from build123d import *

# Parameters (mm, degrees)
BOSS_EXTRUDE1_DEPTH             = 30
CUT_EXTRUDE2_DEPTH              = 9.8
CBORE_FOR_M4_SBHCS1_D           = 4.5
CBORE_FOR_M4_SBHCS1_CBORE_D     = 8.6
CBORE_FOR_M4_SBHCS1_CBORE_DEPTH = 8
F_6_0_6_DIAMETER_HOLE1_D        = 6
SKETCH9_W                       = 7.5
SKETCH9_H                       = 8
CUT_EXTRUDE3_DEPTH              = 19
CUT_EXTRUDE3_DEPTH_BACK         = 19
CHAMFER1_SIZE2                  = 1.68681461
CHAMFER1_SIZE                   = 2
CHAMFER1_EDGE_2_SIZE2           = 1.68681461
CHAMFER1_EDGE_2_SIZE            = 2
F_7_5_7_5_DIAMETER_HOLE1_D      = 7.5
F_7_5_7_5_DIAMETER_HOLE1_DEPTH  = 7
F_7_5_7_5_DIAMETER_HOLE1_TIP    = 2.253227321


with BuildPart() as part:
    # Sketch1 → Boss-Extrude1 (new body)
    with BuildSketch(Plane(origin=(0, 0, 0), x_dir=(1, 0, 0), z_dir=(0, 1, 0))):
        Polygon((-18, 0), (18, 0), (18, 20.8), (14, 24.8), (-14, 24.8), (-18, 20.8), align=None)
    extrude(amount=BOSS_EXTRUDE1_DEPTH)

    # Sketch7 → Cut-Extrude2 (cut)
    with BuildSketch(Plane(origin=(0, 16, 0), x_dir=(1, 0, 0), z_dir=(0, 1, 0))):
        with BuildLine():
            Line((-7, 21.3), (7, 21.3))
            ThreePointArc((7, 21.3), (9.706928791, 20.34103824), (11.206489583, 17.891877451))
            Line((11.206489583, 17.891877451), (15, 0))
            Line((15, 0), (-15, 0))
            Line((-15, 0), (-11.206489583, 17.891877451))
            ThreePointArc((-11.206489583, 17.891877451), (-9.706928791, 20.34103824), (-7, 21.3))
        make_face()
    extrude(amount=CUT_EXTRUDE2_DEPTH, mode=Mode.SUBTRACT)

    # CBORE for M4 SBHCS1 (through all)
    with Locations(Plane(origin=(0, 30, 0), x_dir=(1, 0, 0), z_dir=(0, 1, 0))):
        with Locations((-7, 17), (7, 17)):
            CounterBoreHole(CBORE_FOR_M4_SBHCS1_D / 2, CBORE_FOR_M4_SBHCS1_CBORE_D / 2, CBORE_FOR_M4_SBHCS1_CBORE_DEPTH)

    # Ø6.0 (6) Diameter Hole1 (through all)
    with Locations(Plane(origin=(0, 30, 0), x_dir=(1, 0, 0), z_dir=(0, 1, 0))):
        with Locations((-7, 6), (7, 6)):
            Hole(F_6_0_6_DIAMETER_HOLE1_D / 2)

    # Sketch9 → Cut-Extrude3 (cut, two sides)
    with BuildSketch(Plane(origin=(0, 0, 0), x_dir=(0, 0, -1), z_dir=(1, 0, 0))) as cut_extrude3_sk:
        with Locations((13.75, 20)):
            Rectangle(SKETCH9_W, SKETCH9_H)
    extrude(amount=CUT_EXTRUDE3_DEPTH, mode=Mode.SUBTRACT)
    extrude(cut_extrude3_sk.sketch, amount=-CUT_EXTRUDE3_DEPTH_BACK, mode=Mode.SUBTRACT)

    # Chamfer1
    chamfer1_edges = [part.edges().sort_by_distance(p)[0] for p in [
        (-12.879758328, 20, -10),
    ]]
    chamfer(chamfer1_edges, length=CHAMFER1_SIZE, length2=CHAMFER1_SIZE2)

    # Chamfer1 edge 2
    chamfer1_edge_2_edges = [part.edges().sort_by_distance(p)[0] for p in [
        (12.879758328, 20, -10),
    ]]
    chamfer(chamfer1_edge_2_edges, length=CHAMFER1_EDGE_2_SIZE, length2=CHAMFER1_EDGE_2_SIZE2)

    # Ø7.5 (7.5) Diameter Hole1
    with Locations(Plane(origin=(0, 30, 0), x_dir=(1, 0, 0), z_dir=(0, 1, 0))):
        with Locations((-7, 6), (7, 6)):
            Hole(F_7_5_7_5_DIAMETER_HOLE1_D / 2, depth=F_7_5_7_5_DIAMETER_HOLE1_DEPTH)
            with Locations((0, 0, -(F_7_5_7_5_DIAMETER_HOLE1_DEPTH + F_7_5_7_5_DIAMETER_HOLE1_TIP / 2))):  # 118° drill point
                Cone(0, F_7_5_7_5_DIAMETER_HOLE1_D / 2, F_7_5_7_5_DIAMETER_HOLE1_TIP, mode=Mode.SUBTRACT)


solid = part.part
Design review of the part built by this model. Coordinates are the model's own, in mm. A direction names the side the tool comes from. Give positions to 0.01 mm unless a question says otherwise; leave off trailing zeros. Loops run counter-clockwise (first coordinate to the right, second up) from the corner with the lowest first, then second, coordinate; pieces in that order, holes last. Notation, with made-up numbers: M 60,2 L 92,2 A23 cw 92,13 Z; hole C 33,78 d5. An arc over 180 degrees is marked long. One line per question, with ' | ' between items. Start each with the question number.
1. Add section B-B (z = -16.5). Write out the cut boundary in (x, y), plus the area to 3 significant figures.
2. To check wall thickness, follow L1, parallel to X at y = 7.25, z = -17; L2, parallel to X at y = 26, z = -17; L3, parallel to Z at x = 7, y = 5.75. State the ranges of each line that lie inside material, in increasing order.
3. Insertion check: P1, Ø1, axis at x = -8.5, z = -17.5, coming from the +Y side; P2, Ø7, axis at x = -7, z = -6, coming from the +Y side; P3, Ø1, axis at x = 16, y = 22, coming from the -Z side. Each pin has a flat end and moves straight along its axis. Give the tip position at first contact, or say it passes through.
4. The part is to be moulded in two halves that separate along Y. For faces 1 (the face through (0, 30, -13)), 2 (the face through (0, 16, -11)), 3 (the face through (-9.77, 7.89, -4.85)), say which applies: released by +Y, released by -Y, zero draft, split by the parting line, or undercut.
5. For faces 4 (the face through (-13.973, 21.92, -4.845)), 5 (the face through (0, 15, -24.8)), 6 (the face through (15, 20, -17.5)), 7 (the face through (9.976, 27.871, -3.718)), 8 (the face through (-13.939, 20.056, -9.035)), list the 3-axis set-ups (+Z, -Z, +X, -X, +Y, -Y) from which the entire face can be reached by the end or side of a thin tool; tool diameter is ignored.
6. Add section C-C (x = 8). Write out the cut boundary in (y, z).
7. Add section A-A (y = 17.5). Write out the cut boundary in (x, z).
8. Add section D-D (y = 12.25). Write out the cut boundary in (x, z), plus the area to 3 significant figures.
Worked out:
1) outline: M -18,0 L -9.19,0 L -9.19,16 L -18,16 Z; M -18,24 L -11.5,24 L -11.5,25.8 L -11.27,25.8 L -11.27,30 L -18,30 Z; M -4.81,0 L 4.81,0 L 4.81,16 L -4.81,16 Z; M -2.73,25.8 L 2.73,25.8 L 2.73,30 L -2.73,30 Z; M 9.19,0 L 18,0 L 18,16 L 9.19,16 Z; M 11.27,25.8 L 11.5,25.8 L 11.5,24 L 18,24 L 18,30 L 11.27,30 Z | area: 538 mm²
2) L1: x = -18 to -9.25, -4.75 to 4.75, 9.25 to 18 | L2: x = -18 to -11.3, -2.7 to 2.7, 11.3 to 18 | L3: z = -24.8 to -19.25, -14.75 to -9, -3 to 0
3) P1: passes through | P2: stops at y = 16 | P3: stops at z = -23.3
4) face 1: released by +Y | face 2: undercut | face 3: zero draft
5) face 4: +Z | face 5: -Z, +X, -X, +Y, -Y | face 6: +X, -X | face 7: +Y | face 8: none
6) outline: M 0,-24.8 L 30,-24.8 L 30,-21.18 L 16,-21.18 L 16,-19.02 L 0,-19.02 Z; M 0,-14.98 L 16,-14.98 L 16,-8.83 L 0,-8.83 Z; M 0,-3.17 L 16,-3.17 L 16,0 L 0,0 Z; M 25.8,-12.82 L 30,-12.82 L 30,-9.61 L 25.8,-9.61 Z; M 25.8,-2.39 L 30,-2.39 L 30,0 L 25.8,0 Z
7) outline: M -18,-20.8 L -14,-24.8 L 14,-24.8 L 18,-20.8 L 18,-17.5 L 11.29,-17.5 L 11.21,-17.89 A4.3 cw 7,-21.3 L -7,-21.3 A4.3 cw -11.21,-17.89 L -11.29,-17.5 L -18,-17.5 Z; M -18,-10 L -14.57,-10 L -13.29,-8.04 L -15,0 L -18,0 Z; M 13.29,-8.04 L 14.57,-10 L 18,-10 L 18,0 L 15,0 Z
8) outline: M -18,-20.8 L -14,-24.8 L 14,-24.8 L 18,-20.8 L 18,0 L -18,0 Z; hole C -7,-6 d6; hole C -7,-17 d4.5; hole C 7,-6 d6; hole C 7,-17 d4.5 | area: 788 mm²
